Model file for the job. Use its own axes, mm. A direction names the side the tool comes from. Round coordinates to 2 decimals unless told otherwise and drop trailing zeros. Write each loop counter-clockwise with the first axis right and the second up, starting at its lowest first coordinate (ties: lowest second). Pieces come first, ordered by that corner, then holes.
```python
from build123d import *

# Parameters (mm, degrees)
F1_DEPTH    = 7.5
F3_R        = 5
F4_S5_R     = 4.9585432895
F4_T6_DEPTH = 9
F5_R        = 2


# Not quite as in the source:
# - a fillet or chamfer that OpenCascade refuses, or shapes differently, is made with other operations: its cross-section is extruded or revolved along the edge and cut away or added
# - a feature names something its author has since deleted; it is built from what else it names


with BuildPart() as f1:
    # F0 (on Front) → F1 (new body, symmetric)
    with BuildSketch(Plane.XZ):
        Polygon((-2.3518713359, 1.3106813192), (-2.3518713359, 1.1106813192), (1.854373375, 1.1106813192), (1.854373375, 1.3106813192), (-0.2487489805, 1.3106813192), align=None)
        Polygon((-3.3989118356, -1.6660219789), (3.2814688813, -1.6660219789), (1.8650586641, 1.1106813192), (1.854373375, 1.1106813192), (-2.3518713359, 1.1106813192), align=None)
    extrude(amount=F1_DEPTH, both=True)

    # F0 (on Front) → F2 (revolve)
    with BuildSketch(Plane.XZ):
        Polygon((-7.0862104185, 1.3106813192), (-2.3518713359, 1.3106813192), (-0.2487489805, 1.3106813192), (-0.2487489805, 3.5361030605), (-2.0069789607, 3.5361030605), (-2.0069789607, 37.2762935372), (-5.2072922699, 37.2762935372), (-5.2072922699, 36.3391824067), (-4.6829497442, 35.7728934956), (-4.6829497442, 5.0174454227), align=None)
    revolve(axis=Axis((-0.2487489805, 0, -2.0752633687), (0, 0, -1)))

    # F3
    f3_edges = [f1.edges().sort_by_distance(p)[0] for p in [
        (4.185452, 0, 5.017445),
    ]]
    fillet(f3_edges, radius=F3_R)

    # F4: fillet of radius 2 on 1 edges, made by hand


with BuildPart() as f4_tool2:
    # F4_s3 → F4_t4 (revolve)
    with BuildSketch(Plane.XZ):
        with BuildLine():
            ThreePointArc((-4.6829497442, 34.9891533442), (-4.8208218936, 35.718865526), (-5.2154296124, 36.3479707207))
            Line((-5.2154296124, 36.3479707207), (-4.6829497442, 35.7728934956))
            Line((-4.6829497442, 35.7728934956), (-4.6829497442, 34.9891533442))
        make_face()
    revolve(axis=Axis((-0.2487489805, 0, 35.7728934956), (0, 0, -1)))

    # F4_s5 → F4_t6 (intersect, symmetric)
    with BuildSketch(Plane.XY.offset(35.7)):
        with Locations((-0.2487489805, 0)):
            Circle(F4_S5_R)
    extrude(amount=F4_T6_DEPTH, both=True, mode=Mode.INTERSECT)


with BuildPart() as f1_1:
    add(f1.part)

    # F4_t1: union F4_tool2
    add(f4_tool2.part)

    # F5
    f5_edges = [f1_1.edges().sort_by_distance(p)[0] for p in [
        (-0.248749, 4.958543, 36.339129),
        (-0.248749, -4.958543, 36.339129),
    ]]
    fillet(f5_edges, radius=F5_R)


solid = f1_1.part
```
1) Pull direction Z, two halves, no side cores. Call faces 1 (the face through (0, 0, -1.666)), 2 (the face through (-2.87, -0.11, -0.26)), 3 (the face through (4, 0, 1.311)), 4 (the face through (0, 7, 1.311)): released by +Z, released by -Z, zero draft, split by the parting line, or undercut.
2) Cut at A-A on z = 28. List the corners of the cut face in (x, y).
3) Wall check: probe 1 along Y at (x, z) = (-1.75, 19); probe 2 along Z at (x, y) = (2, -2); probe 3 along Z at (x, y) = (3, 5.25). Give the ranges that are in metal, low to high.
4) Flat gauge pins, fed straight in: pin 1 Ø6 at (x, z) = (0.5, 9.5) entering from -Y; pin 2 Ø8 at (y, z) = (6, 22.5) entering from +X; pin 3 Ø1.1 at (x, y) = (-0.5, -7) entering from +Z. Where does each tip first touch, or does it go through?
5) Which spindle directions (+Z, -Z, +X, -X, +Y, -Y) get a long thin tool onto all of the face, cutting with end or side? Do faces 5 (the face through (-2.63, 3.74, 20.54)), 6 (the face through (-4, 0, 1.311)), 7 (the face through (2.583, -0.105, -0.297)), 8 (the face through (1.147, -1.07, 20.642)). Say none if no direction does.
Result sheet:
1. face 1: released by -Z
1. face 2: undercut
1. face 3: undercut
1. face 4: released by +Z
2. outline: circle Ø8.87 at (-0.25, 0); hole circle Ø3.52 at (-0.25, 0)
3. probe 1: y = -4.17 to -0.92, 0.92 to 4.17
3. probe 2: z = -1.67 to 0.85, 1.31 to 37.28
3. probe 3: z = -1.67 to -1.11, 1.31 to 2.33
4. pin 1: stops at y = -4.43
4. pin 2: stops at x = 3.71
4. pin 3: stops at z = 1.9
5. face 5: none
5. face 6: -X, +Y, -Y
5. face 7: +X, +Y, -Y
5. face 8: +Z
